Autodesk Inventor part; units mm, degrees
ref_plane "YZ Plane" through (0, 0, 0) normal (1, 0, 0) x (0, 1, 0)
ref_plane "XZ Plane" through (0, 0, 0) normal (0, 1, 0) x (-1, 0, 0)
ref_plane "XY Plane" through (0, 0, 0) normal (0, 0, 1) x (1, 0, 0)
sketch "Sketch1" plane through (0, 0, 0) normal (0, 1, 0) x (-1, 0, 0)
  line L0 (7.294, 10.1667) -> (-12.706, 10.1667)
  line L1 (-12.706, 10.1667) -> (-12.706, 0.1667)
  line L2 (-12.706, 0.1667) -> (7.294, 0.1667)
  line L3 (7.294, 0.1667) -> (7.294, 10.1667)
  point P0 (0, 0)
  dimension "d0" = 20
  dimension "d1" = 10
extrude "Extrusion1" add sketch "Sketch1" along normal blind 3
chamfer "Chamfer1" distance 1 angle 45 4 edges at (2.706, 3, 10.1667) (2.706, 0, 10.1667) (2.706, 0, 0.1667) (2.706, 3, 0.1667)
properties part number "lipol-40mAh"
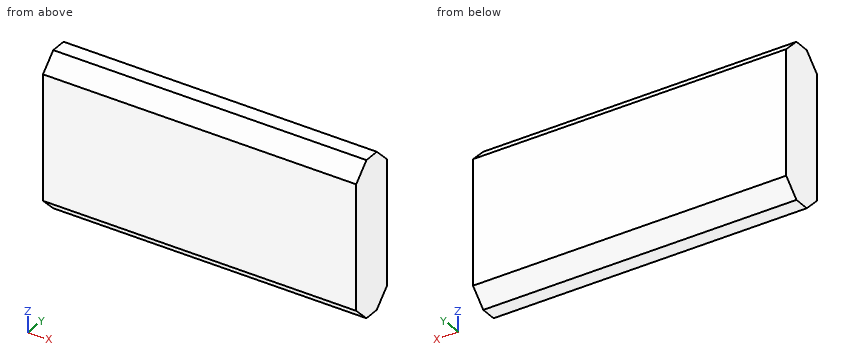
Input: part model. Units: mm. Frame: model coordinates. Coordinates: 2 decimals unless noted, no trailing zeros. Write each loop counter-clockwise with the first axis right and the second up, starting at its lowest first coordinate (ties: lowest second). Pieces come first, ordered by that corner, then holes. Notation, with made-up numbers: (27.5, 29.5) - (85.5, 29.5) arc R19 cw to (85.5, 33.5) - close; hole circle Ø6 at (29.25, 35.5). An arc over 180 degrees is marked (long way). Put each result on its own line as item: value. Start each with the question number.
1) Cut plane A-A (x = -1.5). Return the cut outline in (y, z).
2) Cut plane C-C (y = 2.7). Return the cut outline in (x, z).
3) Cut plane B-B (y = 0.75). Return the cut outline in (x, z).
4) Ray query, L1, parallel to Z at x = -5.75, y = 0.6; L2, parallel to Y at x = 8.75, z = 0.75; L3, parallel to Z at x = -4.75, y = 0.4. Return the intervals inside material, ascending.
Resolved:
1. outline: (0, 1.17) - (1, 0.17) - (2, 0.17) - (3, 1.17) - (3, 9.17) - (2, 10.17) - (1, 10.17) - (0, 9.17) - close
2. outline: (-7.29, 0.87) - (12.71, 0.87) - (12.71, 9.47) - (-7.29, 9.47) - close
3. outline: (-7.29, 0.42) - (12.71, 0.42) - (12.71, 9.92) - (-7.29, 9.92) - close
4. L1: z = 0.57 to 9.77
4. L2: y = 0.42 to 2.58
4. L3: z = 0.77 to 9.57
